Solid Edge part; units mm, degrees
sketch "Sketch1" plane through (0, 0, 0) normal (0, 0, 1) x (1, 0, 0)
  line L0 (-67.5, -72.5) -> (67.5, -72.5)
  line L1 (67.5, -72.5) -> (67.5, 72.5)
  line L2 (67.5, 72.5) -> (-67.5, 72.5)
  line L3 (-67.5, 72.5) -> (-67.5, -72.5)
  dimension "D1" = 67.5
  dimension "D2" = 67.5
extrude "Protrusion1" add sketch "Sketch1" against normal blind 15
hole "Hole_13" at (67.5, -65.5, -8) direction (-1, 0, 0) diameter 3.3 depth 12
hole "Hole1" at (67.5, -49.5, -8) direction (-1, 0, 0) diameter 3.3 depth 12
hole "Hole2" at (67.5, -36.5, -10) direction (-1, 0, 0) diameter 3.3 depth 12
hole "Hole3" at (67.5, 0, -10) direction (-1, 0, 0) diameter 3.3 depth 12
hole "Hole4" at (67.5, 65.5, -10) direction (-1, 0, 0) diameter 3.3 depth 12
hole "Hole_18" at (-67.5, 65.5, -10) direction (1, 0, 0) diameter 3.3 depth 12
hole "Hole5" at (-67.5, 14.5, -10) direction (1, 0, 0) diameter 3.3 depth 12
hole "Hole6" at (-67.5, -36.5, -10) direction (1, 0, 0) diameter 3.3 depth 12
hole "Hole7" at (-67.5, -49.5, -8) direction (1, 0, 0) diameter 3.3 depth 12
hole "Hole8" at (-67.5, -65.5, -8) direction (1, 0, 0) diameter 3.3 depth 12
hole "Hole_23" at (59.5, 39.5, 0) direction (0, 0, -1) diameter 2.5 depth 8
hole "Hole9" at (59.5, 9.5, 0) direction (0, 0, -1) diameter 2.5 depth 8
hole "Hole10" at (59.5, -27.5, 0) direction (0, 0, -1) diameter 2.5 depth 8
hole "Hole11" at (59.5, -57.5, 0) direction (0, 0, -1) diameter 2.5 depth 8
hole "Hole12" at (-57.5, -57.5, 0) direction (0, 0, -1) diameter 2.5 depth 8
hole "Hole13" at (-57.5, -27.5, 0) direction (0, 0, -1) diameter 2.5 depth 8
hole "Hole14" at (-57.5, 9.5, 0) direction (0, 0, -1) diameter 2.5 depth 8
hole "Hole15" at (-57.5, 39.5, 0) direction (0, 0, -1) diameter 2.5 depth 8
hole "Hole16" at (-23.5, 48.5, 0) direction (0, 0, -1) diameter 2.5 depth 8
hole "Hole17" at (11.5, 48.5, 0) direction (0, 0, -1) diameter 2.5 depth 8
hole "Hole_33" at (50, 63.5, -15) direction (0, 0, 1) diameter 4.5 end up to next counterbore diameter 8 counterbore depth 10
hole "Hole18" at (22.5, 63.5, -15) direction (0, 0, 1) diameter 4.5 end up to next counterbore diameter 8 counterbore depth 10
hole "Hole19" at (-12.5, 63.5, -15) direction (0, 0, 1) diameter 4.5 end up to next counterbore diameter 8 counterbore depth 10
hole "Hole20" at (-50, 63.5, -15) direction (0, 0, 1) diameter 4.5 end up to next counterbore diameter 8 counterbore depth 10
fillet "Round_1" radius 1.5 2 edges at (67.5, 72.5, -7.5) (-67.5, 72.5, -7.5)
fillet "Round_2" radius 1.5 2 edges at (-67.5, -72.5, -7.5) (67.5, -72.5, -7.5)
properties material "Acrylic, high impact grade"
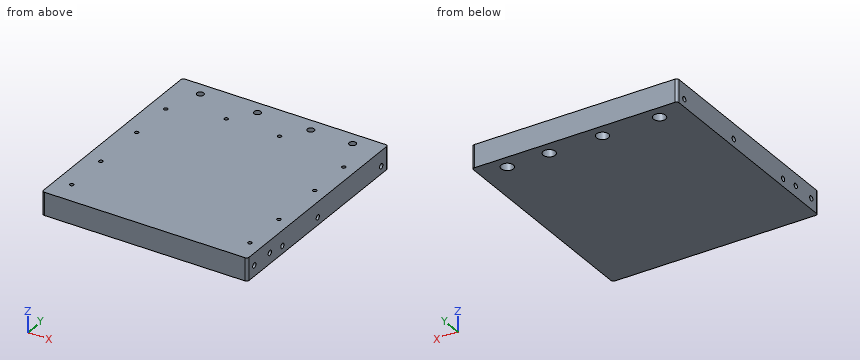
Input: part model. Units: mm. Frame: model coordinates. Round coordinates to 2 decimals unless told otherwise and drop trailing zeros. Order: outer loops, then holes, each group sorted by start corner. A loop starts at its lowest first (then second) coordinate and runs counter-clockwise, first axis right, second up. Notation, with made-up numbers: (63, 24) - (113, 24) arc R8 cw to (113, 28) - close; hole circle Ø5 at (19.5, -17). An arc over 180 degrees is marked (long way). Answer in a Markdown table with one row per item.
Item 1: Section query B-B (y = 0). Return the cut outline in (x, z), then the cut area to 3 significant figures.
Model answer:
| item | result |
|---|---|
| outline | (-67.5, -15) - (67.5, -15) - (67.5, -11.65) - (55.5, -11.65) - (55.5, -8.35) - (67.5, -8.35) - (67.5, 0) - (-67.5, 0) - close |
| area | 1,990 mm² |
Item 2: Line query: line 1 (X direction, y = 63.5, z = -7.5); line 2 (X direction, y = 48.5, z = -2); line 3 (Y direction, x = 22.5, z = -10). Output: solid intervals per line, ascending.
Model answer:
| item | result |
|---|---|
| line 1 | x = -67.5 to -54, -46 to -16.5, -8.5 to 18.5, 26.5 to 46, 54 to 67.5 |
| line 2 | x = -67.5 to -24.75, -22.25 to 10.25, 12.75 to 67.5 |
| line 3 | y = -72.5 to 59.5, 67.5 to 72.5 |
Item 3: Pin query (flat end, axial travel): pin 1 (0.8 mm diameter, centred on x = -57.5, y = -27.5, fed in from +Z); pin 2 (2.5 mm diameter, centred on y = 65.5, z = -10, fed in from -X); pin 3 (2.5 mm diameter, centred on x = 21.5, y = 63, fed in from -Z). Return the tip coordinate at first contact, or that it passes through.
Model answer:
| item | result |
|---|---|
| pin 1 | stops at z = -8 |
| pin 2 | stops at x = -55.5 |
| pin 3 | stops at z = -5 |
Item 4: Section query C-C (y = -65.5). Return the cut outline in (x, z).
Model answer:
| item | result |
|---|---|
| outline | (-67.5, -15) - (67.5, -15) - (67.5, -9.65) - (55.5, -9.65) - (55.5, -6.35) - (67.5, -6.35) - (67.5, 0) - (-67.5, 0) - (-67.5, -6.35) - (-55.5, -6.35) - (-55.5, -9.65) - (-67.5, -9.65) - close |
Item 5: Section query A-A (x = 50). Return the cut outline in (y, z), then the cut area to 3 significant figures.
Model answer:
| item | result |
|---|---|
| outline | (-72.5, -15) - (59.5, -15) - (59.5, -5) - (61.25, -5) - (61.25, 0) - (-72.5, 0) - close; (65.75, -5) - (67.5, -5) - (67.5, -15) - (72.5, -15) - (72.5, 0) - (65.75, 0) - close |
| area | 2,070 mm² |
